Design review of the part built by this model. Coordinates are the model's own, in mm. A direction names the side the tool comes from. Coordinates: 2 decimals unless noted, no trailing zeros. Loops run counter-clockwise (first coordinate to the right, second up) from the corner with the lowest first, then second, coordinate; pieces in that order, holes last. Notation, with made-up numbers: M 89,15 L 144,15 A11 ccw 144,34 Z; hole C -23,12.25 d10. An arc over 180 degrees is marked long. Write item = value, one per line. Start each with the question number.
Solid Edge part; units mm, degrees
sketch "Sketch1" plane through (0, 0, 0) normal (0, -1, 0) x (1, 0, 0)
  line L0 (-20, -20) -> (20, -20)
  line L1 (20, -20) -> (20, 20)
  line L2 (20, 20) -> (-20, 20)
  line L3 (-20, 20) -> (-20, -20)
extrude "Protrusion1" add sketch "Sketch1" along normal mid plane 9
sketch "Sketch2" plane through (0, -4.5, 0) normal (0, -1, 0) x (1, 0, 0)
  line L0 (-15.3, -15.3) -> (15.3, -15.3)
  line L1 (15.3, -15.3) -> (15.3, -9)
  line L2 (10.3, -4) -> (15.3, -9)
  line L3 (10.3, 4) -> (10.3, -4)
  line L4 (10.3, 4) -> (15.3, 9)
  line L5 (15.3, 9) -> (15.3, 15.3)
  line L6 (15.3, 15.3) -> (-15.3, 15.3)
  line L7 (-15.3, 15.3) -> (-15.3, 9)
  line L8 (-10.3, 4) -> (-15.3, 9)
  line L9 (-10.3, 4) -> (-10.3, -4)
  line L10 (-10.3, -4) -> (-15.3, -9)
  line L11 (-15.3, -9) -> (-15.3, -15.3)
extrude "ExtrudedCutout_1" cut sketch "Sketch2" against normal blind 161.5
sketch "Sketch3" plane through (0, -4.5, 2.35) normal (0, -1, 0) x (1, 0, 0)
  line L0 (-12.5, 29.65) -> (-12.5, 17.65)
  line L1 (-12.5, 17.65) -> (12.5, 17.65)
  line L2 (12.5, 29.65) -> (12.5, 17.65)
  arc A0 (12.5, 29.65) -> (-12.5, 29.65) centre (0, 29.65) ccw
extrude "Protrusion2" add sketch "Sketch3" against normal blind 7
sketch "Sketch4" plane through (0, -4.5, 14.6) normal (0, -1, 0) x (1, 0, 0)
  circle A0 centre (0, 17.4) radius 11
extrude "ExtrudedCutout_2" cut sketch "Sketch4" against normal blind 39
sketch "Sketch5" plane through (0, 2.5, 32.25) normal (0, 1, 0) x (0, 0, -1)
  line L0 (0.25, -12.5) -> (12.25, -12.5)
  line L1 (12.25, -12.5) -> (12.25, 12.5)
  line L2 (12.25, 12.5) -> (0.25, 12.5)
  arc A0 (0.25, 12.5) -> (0.25, -12.5) centre (0.25, 0) ccw
extrude "ExtrudedProtrusion_4" add sketch "Sketch5" along normal blind 2
sketch "Sketch6" plane through (0, 4.5, 14.6) normal (0, 1, 0) x (0, 0, -1)
  circle A0 centre (-17.4, 0) radius 4.5
extrude "ExtrudedCutout_3" cut sketch "Sketch6" against normal blind 37
sketch "Sketch7" plane through (0, 0, -15.3) normal (0, 0, 1) x (0, 1, 0)
  line L0 (4.5, 22) -> (4.5, -22)
  line L1 (4.5, -22) -> (-35.5, -22)
  line L2 (-35.5, -22) -> (-35.5, 22)
  line L3 (-35.5, 22) -> (4.5, 22)
  dimension "D1" = 4.5
extrude "Protrusion3" add sketch "Sketch7" against normal blind 30
sketch "Sketch8" plane through (0, -15.5, -45.3) normal (0, 0, -1) x (1, 0, 0)
  line L0 (-20, 20) -> (20, 20)
  line L1 (20, 20) -> (20, -18)
  line L2 (20, -18) -> (-20, -18)
  line L3 (-20, -18) -> (-20, 20)
extrude "ExtrudedCutout_4" cut sketch "Sketch8" against normal blind 28
Q1. Clearance check with flat-ended pins moving along their axes: P1, Ø7, axis at y = 2, z = 13, coming from the -X side; P2, Ø11.5, axis at x = 0, z = 32, coming from the -Y side; P3, Ø2, axis at x = 11, y = -1, coming from the -Z side. State where each tip first meets the part, or that it passes through.
Q2. Mouldability with a two-part tool opening along Z and no side actions: class faces 6 (the face through (12.5, 0, 26)), 7 (the face through (12.8, -0.1, 6.5)), 8 (the face through (0, -16, -17.3)) as released by +Z, released by -Z, zero draft, split by the parting line, or undercut.
Q3. Add section B-B on z = -11.5. State the section outline as (x, y) points, plus the area to 3 significant figures.
Q4. Add section A-A on x = 13.5. State the section outline as (y, z) points, plus the area to 3 significant figures.
Q5. To check wall thickness, follow line 1 (Z direction, x = 0, y = 3.3); line 2 (Z direction, x = 0, y = 1.25); line 3 (X direction, y = -13, z = -35.5). State the ranges of each line that lie inside material, in increasing order. Write a range as from..to.
Q6. Add section C-C on y = -1. Give the number of separate pieces and of enclosed holes in the cut face, plus the area to 3 significant figures.
Q7. Add section D-D on y = -11. State the section outline as (x, z) points, plus the area to 3 significant figures.
Q8. For faces 1 (the face through (-12.8, -0.1, -6.5)), 2 (the face through (-20, -16, -31)), 3 (the face through (-12.5, 0, 26)), 4 (the face through (0, -4.5, 17)), 5 (the face through (0, -16, -15.3)), list the 3-axis set-ups (+Z, -Z, +X, -X, +Y, -Y) from which the entire face can be reached by the end or side of a thin tool; tool diameter is ignored.
Values follow:
q1.P1 = -20
q1.P2 = 2.5
q1.P3 = -17.3
q2.face_6 = zero draft
q2.face_7 = undercut
q2.face_8 = released by -Z
q3.outline = M -20,-4.5 L -15.3,-4.5 L -15.3,4.5 L -20,4.5 Z; M 15.3,-4.5 L 20,-4.5 L 20,4.5 L 15.3,4.5 Z
q3.area = 84.6 mm2
q4.outline = M -35.5,-17.3 L 2.5,-17.3 L 2.5,-45.3 L 4.5,-45.3 L 4.5,-15.3 L -35.5,-15.3 Z; M -4.5,-7.2 L 4.5,-7.2 L 4.5,7.2 L -4.5,7.2 Z; M -4.5,15.3 L 4.5,15.3 L 4.5,20 L -4.5,20 Z
q4.area = 308 mm2
q5.line_1 = -45.3..-15.3, 15.3..27.5, 36.5..44.5
q5.line_2 = -17.3..-15.3, 15.3..21, 43..44.5
q5.line_3 = -22..-20, 20..22
q6.separate_pieces = 1
q6.enclosed_holes = 2
q6.area = 971 mm2
q7.outline = M -22,-45.3 L -20,-45.3 L -20,-17.3 L 20,-17.3 L 20,-45.3 L 22,-45.3 L 22,-15.3 L -22,-15.3 Z
q7.area = 200 mm2
q8.face_1 = +Y, -Y
q8.face_2 = -Z, -Y
q8.face_3 = +Z, -X, +Y, -Y
q8.face_4 = +Z, +X, -X, -Y
q8.face_5 = -Y
